The model under review builds one solid part; all positions refer to its coordinate system, in mm. Face numbers are marked on the shaded views. A direction names the side the tool comes from. Round coordinates to 2 decimals unless told otherwise and drop trailing zeros. Loops run counter-clockwise (first coordinate to the right, second up) from the corner with the lowest first, then second, coordinate; pieces in that order, holes last. Notation, with made-up numbers: M -29,16.25 L -16,16.25 A30 ccw -16,38.25 Z; hole C 41.25,64 d10. An arc over 180 degrees is marked long. Return JSON: item names as keys, results as strings. Group by question number.
Q1. For the marked faces 1, 2 and 3, list the 3-axis set-ups (+Z, -Z, +X, -X, +Y, -Y) from which the entire face can be reached by the end or side of a thin tool; tool diameter is ignored.
Q2. Consider section A-A (y = -1.5). State the section outline as (x, z) points.
Q3. Draft analysis for pull direction X (two halves, no side actions). For the marked faces 4, 5, 6 and 7, state which applies: pulls with the +X half, pulls with the -X half, needs draft (parallel to the pull), parting line crosses it, or undercut.
Q4. Consider section D-D (x = 4). State the section outline as (y, z) points.
Q5. Consider section C-C (z = 5). State the section outline as (x, y) points.
Q6. Clearance check with flat-ended pins moving along their axes: pin 1 Ø2 at (x, z) = (-12, 25) entering from -Y; pin 2 Ø5 at (x, z) = (-13.5, 25.5) entering from +Y; pin 3 Ø10 at (x, z) = (-8, 14.5) entering from +Y; pin 4 Ø5 at (x, y) = (-1, -3) entering from +Z. State where each tip first meets the part, or that it passes through.
Q7. To check wall thickness, follow line 1 along X through (y, z) = (-7.25, 35); line 2 along Z through (x, y) = (-12, -7.75); line 3 along X through (y, z) = (-7.3, 15). State the ranges of each line that lie inside material, in increasing order.
Q8. Consider section B-B (x = -12). State the section outline as (y, z) points, and give its area (4 significant figures).
from build123d import *

# Parameters (mm, degrees)
BOSS_EXTRU_1_DEPTH      = 40
ENL_V_MAT_EXTRU_1_REACH = 14
ESQUISSE2_R             = 1.5
ESQUISSE2_R_2           = 1.25
ESQUISSE3_W             = 15
ESQUISSE3_H             = 20
ENL_V_MAT_EXTRU_2_DEPTH = 6.5
ESQUISSE4_W             = 40
ESQUISSE4_H             = 12
BOSS_EXTRU_2_DEPTH      = 2
CHANFREIN1_SIZE         = 2


with BuildPart() as part:
    # Esquisse1 → Boss.-Extru.1 (new body)
    with BuildSketch(Plane.XY):
        Polygon((5, 0), (20, 0), (20, -12), (-20, -12), (-20, 0), (-5, 0), (-5, -6.5), (5, -6.5), align=None)
    extrude(amount=BOSS_EXTRU_1_DEPTH)

    # Esquisse2 → Enlèv. mat.-Extru.1 (cut, up to next)
    with BuildSketch(Plane(origin=(0, 0, 0), x_dir=(1, 0, 0), z_dir=(0, 1, 0)), mode=Mode.PRIVATE) as enl_v_mat_extru_1_sk1:
        with Locations((-15, -5)):
            Circle(ESQUISSE2_R)
    enl_v_mat_extru_1_tool1 = extrude(enl_v_mat_extru_1_sk1.sketch, amount=-ENL_V_MAT_EXTRU_1_REACH, mode=Mode.PRIVATE) & part.part
    add(enl_v_mat_extru_1_tool1.solids().sort_by_distance((-15, 0, 5))[0], mode=Mode.SUBTRACT)
    # Esquisse2 → Enlèv. mat.-Extru.1 (cut, up to next)
    with BuildSketch(Plane(origin=(0, 0, 0), x_dir=(1, 0, 0), z_dir=(0, 1, 0)), mode=Mode.PRIVATE) as enl_v_mat_extru_1_sk2:
        with Locations((-15, -35)):
            Circle(ESQUISSE2_R)
    enl_v_mat_extru_1_tool2 = extrude(enl_v_mat_extru_1_sk2.sketch, amount=-ENL_V_MAT_EXTRU_1_REACH, mode=Mode.PRIVATE) & part.part
    add(enl_v_mat_extru_1_tool2.solids().sort_by_distance((-15, 0, 35))[0], mode=Mode.SUBTRACT)
    # Esquisse2 → Enlèv. mat.-Extru.1 (cut, up to next)
    with BuildSketch(Plane(origin=(0, 0, 0), x_dir=(1, 0, 0), z_dir=(0, 1, 0)), mode=Mode.PRIVATE) as enl_v_mat_extru_1_sk3:
        with Locations((15, -35)):
            Circle(ESQUISSE2_R)
    enl_v_mat_extru_1_tool3 = extrude(enl_v_mat_extru_1_sk3.sketch, amount=-ENL_V_MAT_EXTRU_1_REACH, mode=Mode.PRIVATE) & part.part
    add(enl_v_mat_extru_1_tool3.solids().sort_by_distance((15, 0, 35))[0], mode=Mode.SUBTRACT)
    # Esquisse2 → Enlèv. mat.-Extru.1 (cut, up to next)
    with BuildSketch(Plane(origin=(0, 0, 0), x_dir=(1, 0, 0), z_dir=(0, 1, 0)), mode=Mode.PRIVATE) as enl_v_mat_extru_1_sk4:
        with Locations((15, -5)):
            Circle(ESQUISSE2_R)
    enl_v_mat_extru_1_tool4 = extrude(enl_v_mat_extru_1_sk4.sketch, amount=-ENL_V_MAT_EXTRU_1_REACH, mode=Mode.PRIVATE) & part.part
    add(enl_v_mat_extru_1_tool4.solids().sort_by_distance((15, 0, 5))[0], mode=Mode.SUBTRACT)
    # Esquisse2 → Enlèv. mat.-Extru.1 (cut, up to next)
    with BuildSketch(Plane(origin=(0, 0, 0), x_dir=(1, 0, 0), z_dir=(0, 1, 0)), mode=Mode.PRIVATE) as enl_v_mat_extru_1_sk5:
        with Locations((-12, -25)):
            Circle(ESQUISSE2_R_2)
    enl_v_mat_extru_1_tool5 = extrude(enl_v_mat_extru_1_sk5.sketch, amount=-ENL_V_MAT_EXTRU_1_REACH, mode=Mode.PRIVATE) & part.part
    add(enl_v_mat_extru_1_tool5.solids().sort_by_distance((-12, 0, 25))[0], mode=Mode.SUBTRACT)
    # Esquisse2 → Enlèv. mat.-Extru.1 (cut, up to next)
    with BuildSketch(Plane(origin=(0, 0, 0), x_dir=(1, 0, 0), z_dir=(0, 1, 0)), mode=Mode.PRIVATE) as enl_v_mat_extru_1_sk6:
        with Locations((-12, -15)):
            Circle(ESQUISSE2_R_2)
    enl_v_mat_extru_1_tool6 = extrude(enl_v_mat_extru_1_sk6.sketch, amount=-ENL_V_MAT_EXTRU_1_REACH, mode=Mode.PRIVATE) & part.part
    add(enl_v_mat_extru_1_tool6.solids().sort_by_distance((-12, 0, 15))[0], mode=Mode.SUBTRACT)
    # Esquisse2 → Enlèv. mat.-Extru.1 (cut, up to next)
    with BuildSketch(Plane(origin=(0, 0, 0), x_dir=(1, 0, 0), z_dir=(0, 1, 0)), mode=Mode.PRIVATE) as enl_v_mat_extru_1_sk7:
        with Locations((12, -25)):
            Circle(ESQUISSE2_R_2)
    enl_v_mat_extru_1_tool7 = extrude(enl_v_mat_extru_1_sk7.sketch, amount=-ENL_V_MAT_EXTRU_1_REACH, mode=Mode.PRIVATE) & part.part
    add(enl_v_mat_extru_1_tool7.solids().sort_by_distance((12, 0, 25))[0], mode=Mode.SUBTRACT)
    # Esquisse2 → Enlèv. mat.-Extru.1 (cut, up to next)
    with BuildSketch(Plane(origin=(0, 0, 0), x_dir=(1, 0, 0), z_dir=(0, 1, 0)), mode=Mode.PRIVATE) as enl_v_mat_extru_1_sk8:
        with Locations((12, -15)):
            Circle(ESQUISSE2_R_2)
    enl_v_mat_extru_1_tool8 = extrude(enl_v_mat_extru_1_sk8.sketch, amount=-ENL_V_MAT_EXTRU_1_REACH, mode=Mode.PRIVATE) & part.part
    add(enl_v_mat_extru_1_tool8.solids().sort_by_distance((12, 0, 15))[0], mode=Mode.SUBTRACT)

    # Esquisse3 → Enlèv. mat.-Extru.2 (cut)
    with BuildSketch(Plane(origin=(0, 0, 0), x_dir=(1, 0, 0), z_dir=(0, 1, 0))):
        with Locations((-12.5, -20)):
            Rectangle(ESQUISSE3_W, ESQUISSE3_H)
        with Locations((12.5, -20)):
            Rectangle(ESQUISSE3_W, ESQUISSE3_H)
    extrude(amount=-ENL_V_MAT_EXTRU_2_DEPTH, mode=Mode.SUBTRACT)

    # Esquisse4 → Boss.-Extru.2 (add)
    with BuildSketch(Plane(origin=(0, 0, 0), x_dir=(-1, 0, 0), z_dir=(0, 0, -1))):
        with Locations((0, -6)):
            Rectangle(ESQUISSE4_W, ESQUISSE4_H)
    extrude(amount=-BOSS_EXTRU_2_DEPTH)

    # Chanfrein1
    chanfrein1_edges = [part.edges().sort_by_distance(p)[0] for p in [
        (-13.25, -12, 25),
        (-13.25, -12, 15),
        (10.75, -12, 25),
        (10.75, -12, 15),
    ]]
    chamfer(chanfrein1_edges, length=CHANFREIN1_SIZE)


solid = part.part
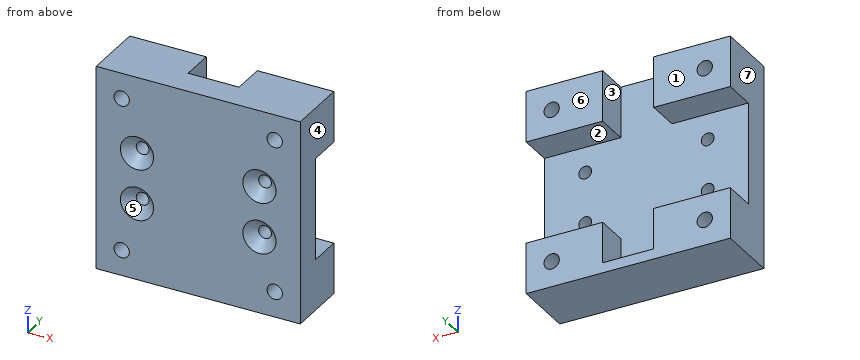
Values:
{
 "1": {"face 1": "+Z, -Z, +X, -X, +Y", "face 2": "+X, -X, +Y", "face 3": "+Z, +Y"},
 "2": {"outline": "M -20,0 L 20,0 L 20,10 L 5,10 L 5,2 L -5,2 L -5,10 L -20,10 Z; M -20,30 L -5,30 L -5,40 L -20,40 Z; M 5,30 L 20,30 L 20,40 L 5,40 Z; hole C -15,5 d3; hole C -15,35 d3; hole C 15,5 d3; hole C 15,35 d3"},
 "3": {"face 4": "pulls with the +X half", "face 5": "undercut", "face 6": "needs draft", "face 7": "pulls with the -X half"},
 "4": {"outline": "M -12,0 L 0,0 L 0,2 L -6.5,2 L -6.5,40 L -12,40 Z"},
 "5": {"outline": "M -20,-12 L -16.5,-12 L -16.5,0 L -20,0 Z; M -13.5,-12 L 13.5,-12 L 13.5,0 L 5,0 L 5,-6.5 L -5,-6.5 L -5,0 L -13.5,0 Z; M 16.5,-12 L 20,-12 L 20,0 L 16.5,0 Z"},
 "6": {"pin 1": "passes through", "pin 2": "stops at y = -6.5", "pin 3": "stops at y = 0", "pin 4": "stops at z = 2"},
 "7": {"line 1": "x = -20 to -16.5, -13.5 to 13.5, 16.5 to 20", "line 2": "z = 0 to 13.75, 16.25 to 23.75, 26.25 to 40", "line 3": "x = -20 to -13.25, -10.75 to 10.75, 13.25 to 20"},
 "8": {"outline": "M -12,0 L 0,0 L 0,10 L -6.5,10 L -6.5,13.75 L -10,13.75 L -12,11.75 Z; M -12,18.25 L -10,16.25 L -6.5,16.25 L -6.5,23.75 L -10,23.75 L -12,21.75 Z; M -12,28.25 L -10,26.25 L -6.5,26.25 L -6.5,30 L 0,30 L 0,40 L -12,40 Z", "area": "314.5 mm2"}
}
